Geometry: final body of the model. Coordinates: model frame, mm. Face numbers are marked on the shaded views. A direction names the side the tool comes from. Coordinates: 2 decimals unless noted, no trailing zeros. Loops run counter-clockwise (first coordinate to the right, second up) from the corner with the lowest first, then second, coordinate; pieces in that order, holes last. Notation, with made-up numbers: (41, -22.5) - (57, -22.5) arc R33 ccw to (57, 8.5) - close; hole circle Ø7 at (-4.75, 55.25). An arc over 180 degrees is marked (long way). Answer in a Markdown table with one row per item.
from build123d import *

# Parameters (mm, degrees)
F1_DEPTH      = 37.5
F3_R          = 3.125
F4_DEPTH      = 37.5
F4_DEPTH_BACK = 37.5
F5_W          = 15.7129609585
F5_H          = 26.9097045064
F5_W_2        = 22.5772851706
F5_H_2        = 27.5291122496
F6_DEPTH      = 71.001
F6_DEPTH_BACK = 5.126
F2_R          = 3
F7_DEPTH      = 71.001


with BuildPart() as f1:
    # F0 (on Front) → F1 (new body, symmetric)
    with BuildSketch(Plane.XZ):
        with BuildLine():
            ThreePointArc((64.3155620097, -9.4078947368), (0, -65), (-64.3155620097, -9.4078947368))
            ThreePointArc((-64.3155620097, -9.4078947368), (-68.0064440401, -2.6779462302), (-75.1997340421, 0))
            Line((-75.1997340421, 0), (-110, 0))
            Line((-110, 0), (-110, -6))
            Line((-110, -6), (-75.1997340421, -6))
            ThreePointArc((-75.1997340421, -6), (-71.9300567685, -7.2172482865), (-70.2523831183, -10.2763157895))
            ThreePointArc((-70.2523831183, -10.2763157895), (0, -71), (70.2523831183, -10.2763157895))
            ThreePointArc((70.2523831183, -10.2763157895), (71.9300567685, -7.2172482865), (75.1997340421, -6))
            Line((75.1997340421, -6), (110, -6))
            Line((110, -6), (110, 0))
            Line((110, 0), (75.1997340421, 0))
            ThreePointArc((75.1997340421, 0), (68.0064440401, -2.6779462302), (64.3155620097, -9.4078947368))
        make_face()
    extrude(amount=F1_DEPTH, both=True)

    # F3 (on Front) → F4 (join, two sides)
    with BuildSketch(Plane.XZ) as f4_sk:
        with BuildLine():
            ThreePointArc((110, -3.971), (110.4913325801, -3.253734436), (111.3376547749, -3.4527729648))
            ThreePointArc((111.3376547749, -3.4527729648), (119.9038999403, 1.851415772), (110, 0))
            Line((110, 0), (110, -3.971))
        make_face()
        with Locations((115.125, 0)):
            Circle(F3_R, mode=Mode.SUBTRACT)
    extrude(amount=F4_DEPTH)
    extrude(f4_sk.sketch, amount=-F4_DEPTH_BACK)

    # F5 (on Top) → F6 (cut, two sides)
    with BuildSketch(Plane.XY) as f6_sk:
        with Locations((117.8564804792, -25.9548522532)):
            Rectangle(F5_W, F5_H)
        with Locations((121.2886425853, 26.2645561248)):
            Rectangle(F5_W_2, F5_H_2)
    extrude(amount=-F6_DEPTH, mode=Mode.SUBTRACT)
    extrude(f6_sk.sketch, amount=F6_DEPTH_BACK, mode=Mode.SUBTRACT)

    # F2 (on face) → F7 (cut, through all)
    with BuildSketch(Plane.XY):
        with Locations((-90, 17.5)):
            Circle(F2_R)
        with Locations((-90, -17.5)):
            Circle(F2_R)
    extrude(amount=-F7_DEPTH, mode=Mode.SUBTRACT)


solid = f1.part
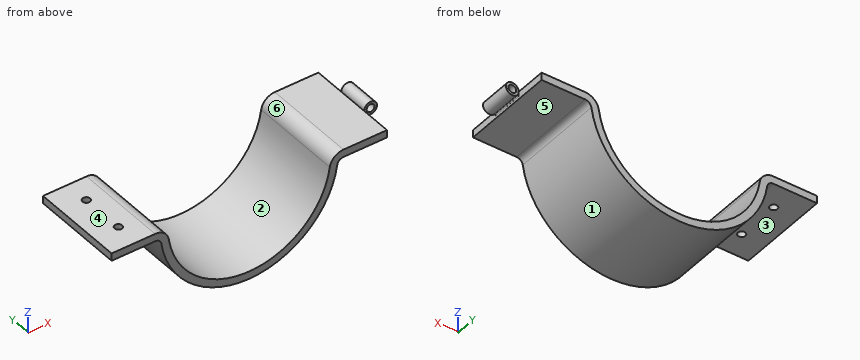
(1) Cut plane B-B on x = -90. Output: boundary loops of the cut face in (y, z), then the cut area to 3 significant figures.
Verdict:
| item | result |
|---|---|
| outline | (-37.5, -6) - (-20.5, -6) - (-20.5, 0) - (-37.5, 0) - close; (-14.5, -6) - (14.5, -6) - (14.5, 0) - (-14.5, 0) - close; (20.5, -6) - (37.5, -6) - (37.5, 0) - (20.5, 0) - close |
| area | 378 mm² |
(2) First-contact query: pin 1 Ø8 at (x, y) = (-90, -17.5) entering from -Z; pin 2 Ø10 at (y, z) = (-4.5, -18) entering from +X; pin 3 Ø2 at (x, y) = (-2, -9.5) entering from -Z; pin 4 Ø5 at (x, z) = (115.125, 0) entering from +Y (3 decimals). Flat tips, straight axial feed; report the tip coordinate or a pass-through.
Verdict:
| item | result |
|---|---|
| pin 1 | stops at z = -6 |
| pin 2 | stops at x = 69.8 |
| pin 3 | stops at z = -70.99 |
| pin 4 | passes through |
(3) Cut plane A-A on y = 17.5. Output: boundary loops of the cut face in (x, z), then the cut area to 3 significant figures.
Verdict:
| item | result |
|---|---|
| outline | (-110, -6) - (-93, -6) - (-93, 0) - (-110, 0) - close; (-87, -6) - (-75.2, -6) arc R5 cw to (-70.25, -10.28) arc R71 ccw to (70.25, -10.28) arc R5 cw to (75.2, -6) - (110, -6) - (110, 0) - (75.2, 0) arc R11 ccw to (64.32, -9.41) arc R65 cw to (-64.32, -9.41) arc R11 ccw to (-75.2, 0) - (-87, 0) - close |
| area | 1,680 mm² |
(4) Access query for the marked faces 4, 5 and 6. Directions: +Z, -Z, +X, -X, +Y, -Y. A direction counts if a zero-diameter tool reaches every point of the face in a straight line with its end or side. Return the directions, or none.
Verdict:
| item | result |
|---|---|
| face 4 | +Z, -X, +Y, -Y |
| face 5 | -Z, +X, +Y, -Y |
| face 6 | +Z, +Y, -Y |
(5) Cut plane C-C on z = -47. Output: boundary loops of the cut face in (x, y).
Verdict:
| item | result |
|---|---|
| outline | (-53.22, -37.5) - (-44.9, -37.5) - (-44.9, 37.5) - (-53.22, 37.5) - close; (44.9, -37.5) - (53.22, -37.5) - (53.22, 37.5) - (44.9, 37.5) - close |
(6) Cut plane D-D on y = 3.5. Output: boundary loops of the cut face in (x, z) (3 decimals).
Verdict:
| item | result |
|---|---|
| outline | (-110, -6) - (-75.2, -6) arc R5 cw to (-70.252, -10.276) arc R71 ccw to (70.252, -10.276) arc R5 cw to (75.2, -6) - (110, -6) - (110, -3.971) arc R0.769 cw to (111.338, -3.453) arc R5.125 ccw (long way) to (110, 0) - (75.2, 0) arc R11 ccw to (64.316, -9.408) arc R65 cw to (-64.316, -9.408) arc R11 ccw to (-75.2, 0) - (-110, 0) - close; hole circle Ø6.25 at (115.125, 0) |
(7) Ray query, probe 1 along Y at (x, z) = (-90, -2.5); probe 2 along Z at (x, y) = (87, -34); probe 3 along X at (y, z) = (-25.5, -14.5). Return the intervals inside material, ascending.
Verdict:
| item | result |
|---|---|
| probe 1 | y = -37.5 to -20.5, -14.5 to 14.5, 20.5 to 37.5 |
| probe 2 | z = -6 to 0 |
| probe 3 | x = -69.5 to -63.36, 63.36 to 69.5 |
(8) Pull-direction query (X, two-part tool) for the marked faces 1, 2 and 3; classes: pulls with the +X half, pulls with the -X half, needs draft (parallel to the pull), parting line crosses it, or undercut.
Verdict:
| item | result |
|---|---|
| face 1 | parting line crosses it |
| face 2 | undercut |
| face 3 | needs draft |
